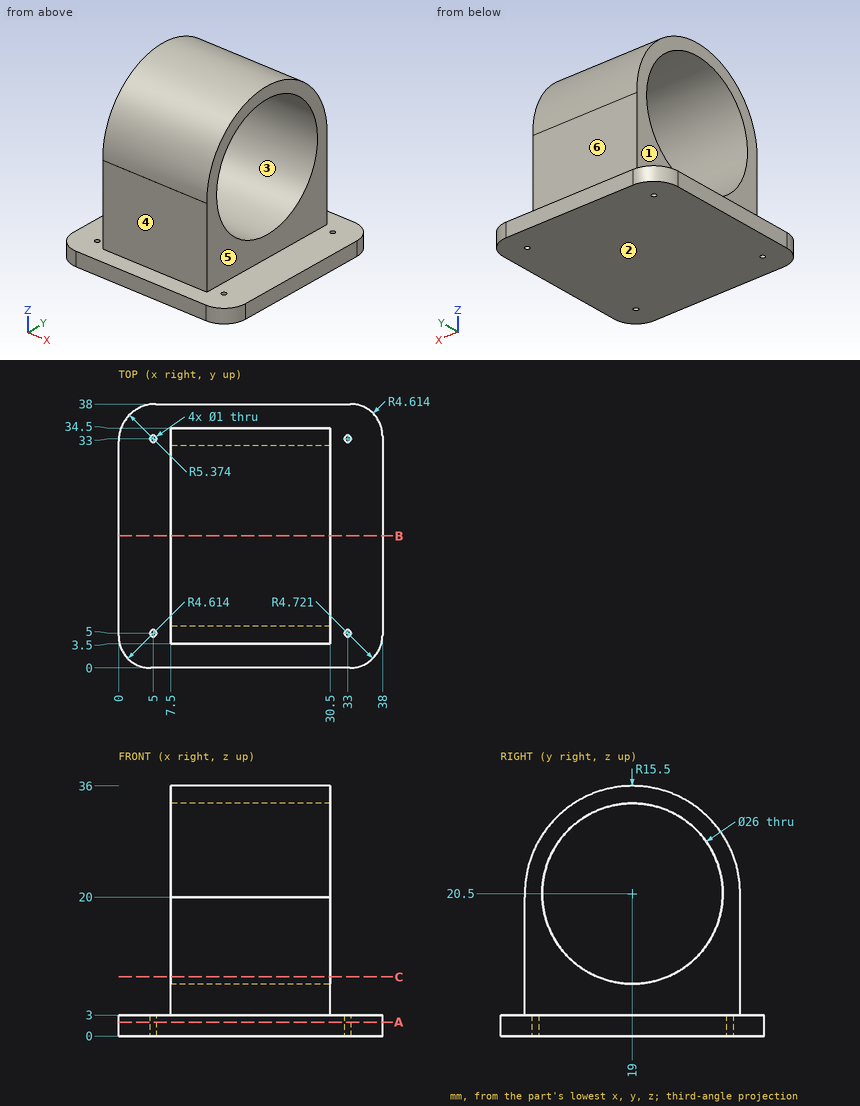
Answer from the drawing. Dimensions are ordinates in mm from the lowest x, y and z of the part. A direction names the side the tool comes from. Round coordinates to 2 decimals unless told otherwise and drop trailing zeros. Loops run counter-clockwise (first coordinate to the right, second up) from the corner with the lowest first, then second, coordinate; pieces in that order, holes last.
(1) The mould has two halves that part along Z. Classify the marked faces 1, 2 and 3: pulls with the +Z half, pulls with the -Z half, needs draft (parallel to the pull), parting line crosses it, or undercut.
Computed values:
face 1: needs draft
face 2: pulls with the -Z half
face 3: undercut
(2) Find the intervals of material crossed by L1, parallel to Y at x = 33, z = 1; L2, parallel to Z at x = 16, y = 19; L3, parallel to Z at x = 36.5, y = 9.5, in increasing order.
Computed values:
L1: y = 0 to 4.5, 5.5 to 32.5, 33.5 to 38
L2: z = 0 to 7.5, 33.5 to 36
L3: z = 0 to 3
(3) For the marked faces 4, 5 and 6, determine the directions among +Z, -Z, +X, -X, +Y, -Y from which every point of the face is accessible in a straight line to the end or side of a thin tool.
Computed values:
face 4: +Z, +X, -X, -Y
face 5: +Z, +X, +Y, -Y
face 6: +Z, +X, -X, +Y
(4) Each of these flat-tipped pins is pushed along its axis until it touches: P1, Ø1, axis at x = 14.5, z = 8.5, coming from the -Y side; P2, Ø1, axis at y = 4, z = 4, coming from the +X side; P3, Ø3, axis at x = 28, z = 25.5, coming from the -Y side; P4, Ø12, axis at y = 19, z = 15.5, coming from the -X side. Where does it stop, or does it pass through?
Computed values:
P1: stops at y = 3.5
P2: stops at x = 30.5
P3: stops at y = 3.9
P4: passes through
(5) The part is cut by section C-C, the plane z = 8.5. Give the vertices of the cut face in (x, y).
Computed values:
outline: (7.5, 3.5) - (30.5, 3.5) - (30.5, 14) - (7.5, 14) - close; (7.5, 24) - (30.5, 24) - (30.5, 34.5) - (7.5, 34.5) - close
(6) The part is cut by section A-A, the plane z = 2. Give the vertices of the cut face in (x, y) (1 decimal).
Computed values:
outline: (0, 4.6) arc R4.6 ccw to (4.6, 0) - (33.3, 0) arc R4.7 ccw to (38, 4.7) - (38, 33.4) arc R4.6 ccw to (33.4, 38) - (5.4, 38) arc R5.4 ccw to (0, 32.6) - close; hole circle Ø1 at (5, 5); hole circle Ø1 at (5, 33); hole circle Ø1 at (33, 5); hole circle Ø1 at (33, 33)
(7) The part is cut by section B-B, the plane y = 19. Give the vertices of the cut face in (x, z), and give its area (3 significant figures).
Computed values:
outline: (0, 0) - (38, 0) - (38, 3) - (30.5, 3) - (30.5, 7.5) - (7.5, 7.5) - (7.5, 3) - (0, 3) - close; (7.5, 33.5) - (30.5, 33.5) - (30.5, 36) - (7.5, 36) - close
area: 275 mm2
